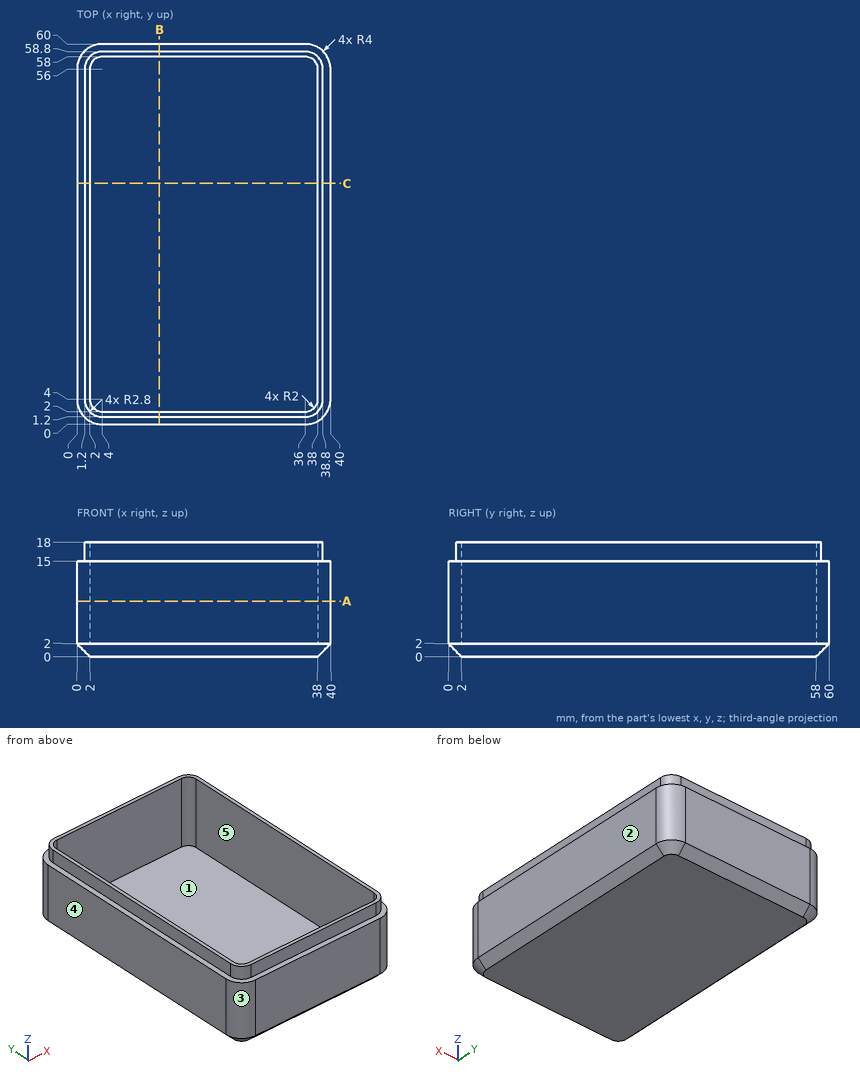
Verification items for this drawing (mm, ordinates from the low corner). A direction names the side the tool comes from. Coordinates: 2 decimals unless noted, no trailing zeros. Order: outer loops, then holes, each group sorted by start corner. A loop starts at its lowest first (then second) coordinate and runs counter-clockwise, first axis right, second up. Notation, with made-up numbers: M 33.5,51 L 85.5,51 A15 ccw 85.5,80 Z; hole C 87.5,-28.75 d4. An arc over 180 degrees is marked long. Answer as a JSON object with one key per item and string values.
Q1. Cross-section at A-A on z = 8.75. Record the cut outline in (x, y), and give its area (3 significant figures).
Results are:
{"outline": "M 0,4 A4 ccw 4,0 L 36,0 A4 ccw 40,4 L 40,56 A4 ccw 36,60 L 4,60 A4 ccw 0,56 Z; hole M 2,4 A2 ccw 4,2 L 36,2 A2 ccw 38,4 L 38,56 A2 ccw 36,58 L 4,58 A2 ccw 2,56 Z", "area": "374 mm²"}
Q2. Cross-section at C-C on y = 38. Record the cut outline in (x, z), and give its area (3 significant figures).
Results are:
{"outline": "M 0,2 L 2,0 L 38,0 L 40,2 L 40,15 L 38.8,15 L 38.8,18 L 38,18 L 38,2 L 2,2 L 2,18 L 1.2,18 L 1.2,15 L 0,15 Z", "area": "133 mm²"}
Q3. Scan lines: line 1 (Y direction, x = 12, z = 8.5); line 2 (X direction, y = 30.5, z = 14.5); line 3 (Y direction, x = 27, z = 16.75). Record each from-to range of solid material in increasing order.
Results are:
{"line 1": "y = 0 to 2, 58 to 60", "line 2": "x = 0 to 2, 38 to 40", "line 3": "y = 1.2 to 2, 58 to 58.8"}
Q4. Depth check by flat-ended pin: pin 1 Ø3 at (x, y) = (16.5, 37) entering from +Z; pin 2 Ø0.9 at (y, z) = (39, 16.5) entering from +X; pin 3 Ø0.9 at (x, z) = (13, 17) entering from -Y. Enter the tip coordinate at first touch or a pass-through.
Results are:
{"pin 1": "stops at z = 2", "pin 2": "stops at x = 38.8", "pin 3": "stops at y = 1.2"}
Q5. Release check for a two-part mould opening along Y. For the marked faces 1, 2 and 3 record: released by +Y, released by -Y, zero draft, split by the parting line, or undercut.
Results are:
{"face 1": "undercut", "face 2": "zero draft", "face 3": "released by -Y"}
Q6. Cross-section at B-B on x = 13. Record the cut outline in (y, z).
Results are:
{"outline": "M 0,2 L 2,0 L 58,0 L 60,2 L 60,15 L 58.8,15 L 58.8,18 L 58,18 L 58,2 L 2,2 L 2,18 L 1.2,18 L 1.2,15 L 0,15 Z"}
Q7. Tool access check on the marked faces 4 and 5. Record the directions out of +Z, -Z, +X, -X, +Y, -Y that give a thin tool (end or side, any length) a straight path to the whole face; none if there is none.
Results are:
{"face 4": "+Z, -Z, -X, +Y, -Y", "face 5": "+Z"}
